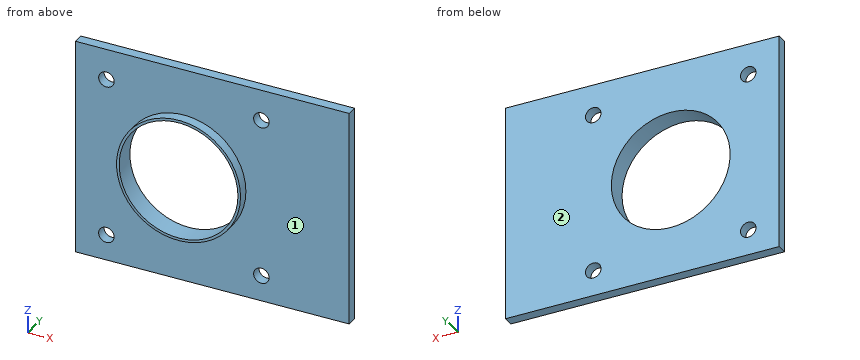
Autodesk Inventor part; units mm, degrees
ref_plane "YZ Plane" through (0, 0, 0) normal (1, 0, 0) x (0, 1, 0)
ref_plane "XZ Plane" through (0, 0, 0) normal (0, 1, 0) x (-1, 0, 0)
ref_plane "XY Plane" through (0, 0, 0) normal (0, 0, 1) x (1, 0, 0)
sketch "Sketch1" plane through (0, 0, 0) normal (0, 1, 0) x (-1, 0, 0)
  line L0 (0, 0) -> (32, 0)
  circle A0 centre (32, 0) radius 12
  line L1 (53, 21) -> (11, 21)
  line L2 (11, 21) -> (11, -21)
  line L3 (11, -21) -> (53, -21)
  line L4 (53, -21) -> (53, 21)
  line L5 (53, 21) -> (11, -21) construction
  line L6 (11, 21) -> (53, -21) construction
  circle A1 centre (47, 15) radius 1.5
  circle A2 centre (47, -16) radius 1.5
  line L7 (32, 0) -> (32, 21)
  circle A3 centre (17, 15) radius 1.5
  circle A4 centre (17, -16) radius 1.5
  line L8 (11, 21) -> (0, 21)
  line L9 (0, 21) -> (0, -21)
  line L10 (0, -21) -> (11, -21)
  dimension "d0" = 32
  dimension "d1" = 24
  dimension "d2" = 42
  dimension "d3" = 42
  dimension "d4" = 3
  dimension "d5" = 3
  dimension "d6" = 31
  dimension "d7" = 15
  dimension "d8" = 15
  dimension "d14" = 11
extrude "Extrusion1" add sketch "Sketch1" along normal blind 2 contours L9 L8 L2 L0 | L0 L2 L10 L9 | L2 L1 L7 A0 L0 | L0 A0 L7 L1 L4 L3 L2
sketch "Sketch2" plane through (0, 0, 0) normal (0, -1, 0) x (1, 0, 0)
  line L0 (-53, -21) -> (-53, 21)
  circle A0 centre (-17, 15) radius 1.5
  circle A1 centre (-32, 0) radius 12
  circle A2 centre (-17, -16) radius 1.5
  circle A3 centre (-47, 15) radius 1.5
  circle A4 centre (-47, -16) radius 1.5
  circle A5 centre (-32, 0) radius 11.5
  line L1 (0, -21) -> (-53, -21)
  line L2 (0, 21) -> (0, -21)
  line L3 (-53, 21) -> (0, 21)
  point P0 (0, 0)
  dimension "d11" = 23
extrude "Extrusion2" add sketch "Sketch2" along normal mid plane 4 contours A1
properties part number "2_3DPrint"
The listing builds one solid part. Answer for the finished solid, in the listing's coordinates (mm). Face numbers are marked on the shaded views. A direction names the side the tool comes from. Round coordinates to 2 decimals unless told otherwise and drop trailing zeros. Order: outer loops, then holes, each group sorted by start corner. A loop starts at its lowest first (then second) coordinate and runs counter-clockwise, first axis right, second up. Notation, with made-up numbers: (57.5, 73.25) -> (66.5, 73.25) arc R20 ccw to (66.5, 81.25) -> close; hole circle Ø10 at (79.5, 82.5). An arc over 180 degrees is marked (long way). Write each question's results on one line, items separated by ' | '. Start each with the question number.
Q1. Find section D-D (x = -17). Determine the outline of the cut face in (y, z).
Q2. Straight lines are drawn through the part: probe 1 along Z at (x, y) = (-47, 0.85); probe 2 along Z at (x, y) = (-16.5, 0.35); probe 3 along Z at (x, y) = (-32.5, -1). For each, find the intervals that lie inside material, in ascending order. Write a range as from..to.
Q3. Find section A-A (z = 0). Determine the outline of the cut face in (x, y).
Q4. Find section C-C (z = -16). Determine the outline of the cut face in (x, y), then the cut area to 3 significant figures.
Q5. Which of the six approach directions +Z, -Z, +X, -X, +Y, -Y give full straight-line access (tool end or side, diameter ignored) to the marked faces 1 and 2?
Q6. Find section B-B (x = -32). Determine the outline of the cut face in (y, z).
Q7. This flat-tipped pin is pushed along its axis until it touches: pin 1 (1 mm diameter, centred on x = -16.5, z = -9.5, fed in from -Y). Where does it stop, or does it pass through?
Worked answers:
1) outline: (0, -21) -> (2, -21) -> (2, -17.5) -> (0, -17.5) -> close; (0, -14.5) -> (2, -14.5) -> (2, 13.5) -> (0, 13.5) -> close; (0, 16.5) -> (2, 16.5) -> (2, 21) -> (0, 21) -> close
2) probe 1: z = -21..-17.5, -14.5..13.5, 16.5..21 | probe 2: z = -21..-17.41, -14.59..13.59, 16.41..21 | probe 3: z = -11.99..-11.49, 11.49..11.99
3) outline: (-53, 0) -> (-44, 0) -> (-44, -2) -> (-43.5, -2) -> (-43.5, 2) -> (-53, 2) -> close; (-20.5, -2) -> (-20, -2) -> (-20, 0) -> (0, 0) -> (0, 2) -> (-20.5, 2) -> close
4) outline: (-53, 0) -> (-48.5, 0) -> (-48.5, 2) -> (-53, 2) -> close; (-45.5, 0) -> (-18.5, 0) -> (-18.5, 2) -> (-45.5, 2) -> close; (-15.5, 0) -> (0, 0) -> (0, 2) -> (-15.5, 2) -> close | area: 94.0 mm2
5) face 1: -Y | face 2: +Z, -Z, +X, -X, +Y
6) outline: (-2, -12) -> (0, -12) -> (0, -21) -> (2, -21) -> (2, -11.5) -> (-2, -11.5) -> close; (-2, 11.5) -> (2, 11.5) -> (2, 21) -> (0, 21) -> (0, 12) -> (-2, 12) -> close
7) pin 1: stops at y = 0
